```python
from build123d import *

# Parameters (mm, degrees)
SKETCH_1_W               = 20
SKETCH_1_H               = 10
EXTRUDE_1_DEPTH          = 9
CUT_EXTRUDE_3_DEPTH      = 9
CUT_EXTRUDE_4_DEPTH      = 18.52868966
CUT_EXTRUDE_4_DEPTH_BACK = 9
EXTRUDE_2_DEPTH          = 9
EXTRUDE_3_DEPTH          = 9
SKETCH_10_W              = 8
SKETCH_10_H              = 13
CUT_EXTRUDE_5_DEPTH      = 9
SKETCH_12_W              = 2.5
SKETCH_12_H              = 12
CUT_EXTRUDE_6_DEPTH      = 9
SKETCH_13_W              = 2.5
SKETCH_13_H              = 7.75
CUT_EXTRUDE_7_DEPTH      = 9
CUT_EXTRUDE_8_DEPTH      = 9
CUT_EXTRUDE_9_DEPTH      = 9
SKETCH_18_R              = 0.25
CUT_EXTRUDE_12_DEPTH     = 18.568302001
SKETCH_26_R              = 0.25
CUT_EXTRUDE_16_DEPTH     = 19.638541659


with BuildPart() as part:
    # 草图1 → 凸台-拉伸1 (new body)
    with BuildSketch(Plane(origin=(0, 0, 0), x_dir=(0, 0, -1), z_dir=(1, 0, 0))):
        with Locations((-3.964524465, 0.58990319)):
            Rectangle(SKETCH_1_W, SKETCH_1_H)
    extrude(amount=EXTRUDE_1_DEPTH)

    # 草图2 → 切除-拉伸3 (cut)
    with BuildSketch(Plane(origin=(9, 0, 0), x_dir=(0, 0, -1), z_dir=(1, 0, 0))):
        Polygon((0.035475535, -0.41009681), (-3.964524465, -4.41009681), (6.035475535, -4.41009681), (6.035475535, -0.410096535), align=None)
    extrude(amount=-CUT_EXTRUDE_3_DEPTH, mode=Mode.SUBTRACT)

    # 草图6 → 切除-拉伸4 (cut, two sides: drawn at the far end of the back side and taken through both)
    with BuildSketch(Plane(origin=(9, 0, 0), x_dir=(0, 0, -1), z_dir=(1, 0, 0)).offset(-CUT_EXTRUDE_4_DEPTH_BACK)):
        Polygon((-66.684543288, -0.910096672), (-13.964524465, -0.910096672), (-3.964524465, -0.910096672), (0.035475535, 3.089903328), (6.035475535, 3.089903328), (58.755494358, 3.089903328), (55.394957379, 108.476374614), (-70.045080267, 104.476374614), align=None)
    extrude(amount=CUT_EXTRUDE_4_DEPTH + CUT_EXTRUDE_4_DEPTH_BACK, mode=Mode.SUBTRACT)

    # 草图8 → 凸台-拉伸2 (add)
    with BuildSketch(Plane(origin=(9, 0, 0), x_dir=(0, 0, -1), z_dir=(1, 0, 0))):
        with BuildLine():
            Line((-13.964524465, -4.41009681), (-13.964524465, -0.910096672))
            ThreePointArc((-13.964524465, -0.910096672), (-15.714524534, -2.660096741), (-13.964524465, -4.41009681))
        make_face()
    extrude(amount=-EXTRUDE_2_DEPTH)

    # 草图9 → 凸台-拉伸3 (add)
    with BuildSketch(Plane(origin=(9, 0, 0), x_dir=(0, 0, -1), z_dir=(1, 0, 0))):
        with BuildLine():
            Line((6.035475535, -0.410096672), (6.035475535, 3.089903328))
            ThreePointArc((6.035475535, 3.089903328), (7.785475535, 1.339903328), (6.035475535, -0.410096672))
        make_face()
    extrude(amount=-EXTRUDE_3_DEPTH)

    # 草图10 → 切除-拉伸5 (cut)
    with BuildSketch(Plane(origin=(0, -0.910096672, 0), x_dir=(1, 0, 0), z_dir=(0, 1, 0))):
        with Locations((4.5, -10.464524465)):
            Rectangle(SKETCH_10_W, SKETCH_10_H)
    extrude(amount=-CUT_EXTRUDE_5_DEPTH, mode=Mode.SUBTRACT)

    # 草图12 → 切除-拉伸6 (cut)
    with BuildSketch(Plane(origin=(0, 3.089903328, 0), x_dir=(1, 0, 0), z_dir=(0, 1, 0))):
        with Locations((7.75, 6.035475535)):
            Rectangle(SKETCH_12_W, SKETCH_12_H)
    extrude(amount=-CUT_EXTRUDE_6_DEPTH, mode=Mode.SUBTRACT)

    # 草图13 → 切除-拉伸7 (cut)
    with BuildSketch(Plane(origin=(0, 3.089903328, 0), x_dir=(1, 0, 0), z_dir=(0, 1, 0))):
        with Locations((1.25, 3.910475535)):
            Rectangle(SKETCH_13_W, SKETCH_13_H)
    extrude(amount=-CUT_EXTRUDE_7_DEPTH, mode=Mode.SUBTRACT)

    # 草图14 → 切除-拉伸8 (cut)
    with BuildSketch(Plane(origin=(0, 1.527213896, 1.527213896), x_dir=(1, 0, 0), z_dir=(0, 0.7071067811865477, 0.7071067811865475))):
        Polygon((2.5, 2.209976588), (0, -3.446877662), (-6.872938914, -0.617067375), (-4.372938914, 5.039786874), align=None)
    extrude(amount=-CUT_EXTRUDE_8_DEPTH, mode=Mode.SUBTRACT)

    # 草图15 → 切除-拉伸9 (cut)
    with BuildSketch(Plane(origin=(0, 1.527213896, 1.527213896), x_dir=(1, 0, 0), z_dir=(0, 0.7071067811865477, 0.7071067811865475))):
        Polygon((6.5, 2.209976588), (9, -3.446877662), (12.673354488, 0), (10.173354488, 5.656854249), align=None)
    extrude(amount=-CUT_EXTRUDE_9_DEPTH, mode=Mode.SUBTRACT)

    # 草图18 → 切除-拉伸12 (cut, through all)
    with BuildSketch(Plane(origin=(6.5, 0, 0), x_dir=(0, 0, -1), z_dir=(1, 0, 0))):
        with Locations((6.035475535, 1.339903328)):
            Circle(SKETCH_18_R)
    extrude(amount=-CUT_EXTRUDE_12_DEPTH, mode=Mode.SUBTRACT)

    # 草图26 → 切除-拉伸16 (cut, through all)
    with BuildSketch(Plane.ZY):
        with Locations((13.964524465, -2.660096741)):
            Circle(SKETCH_26_R)
    extrude(amount=-CUT_EXTRUDE_16_DEPTH, mode=Mode.SUBTRACT)


solid = part.part
```
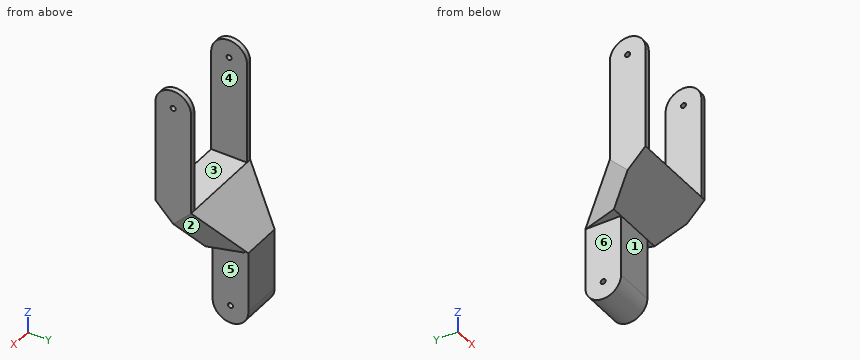
Part model, mm, in its own coordinate system. Face numbers are marked on the shaded views. A direction names the side the tool comes from. Round coordinates to 2 decimals unless told otherwise and drop trailing zeros. Loops run counter-clockwise (first coordinate to the right, second up) from the corner with the lowest first, then second, coordinate; pieces in that order, holes last. Notation, with made-up numbers: (24, -9) -> (66, -9) arc R23 cw to (66, 18) -> close; hole circle Ø2 at (-36, -32.5). An arc over 180 degrees is marked (long way). Use CSV: the item, a comma, the result in double quotes. Start each with the question number.
1) Cut at A-A, the plane z = 6. Write the cut outline in (x, y).
2) Cut at B-B, the plane x = 2.75. Write the cut outline in (y, z).
3) Which spindle directions (+Z, -Z, +X, -X, +Y, -Y) get a long thin tool onto all of the face, cutting with end or side? Do the marked faces 4, 5 and 6. Say none if no direction does.
4) Wall check: L1, parallel to X at y = -3.75, z = 11.5; L2, parallel to Y at x = 4.5, z = -3.5; L3, parallel to X at y = -0.5, z = 3.5. Give the ranges that are in metal, low to high. Write a range as [from, to].
5) Cut at D-D, the plane x = 6.75. Write the cut outline in (y, z), plus the area to 3 significant figures.
6) Pull direction X, two halves, no side cores. Call the marked faces 1, 2 and 3: +X half, -X half, draft (parallel to the pull), parting line (faces both ways), or undercut.
7) Drop flat-ended pins along their axis: P1, Ø2, axis at x = 4.5, z = -3, coming from the -Y side; P2, Ø0.9, axis at x = 7, y = 1, coming from the -Z side; P3, Ø1, axis at x = 2.5, y = 0.5, coming from the -Z side. Give the stop position or say it passes through.
8) Cut at C-C, the plane y = 0. Write the cut outline in (x, z).
Determined:
1,outline,"(0, -4.41) -> (0.5, -4.41) -> (0.5, -0.91) -> (0, -0.91) -> close; (8.5, -4.41) -> (9, -4.41) -> (9, -0.91) -> (8.5, -0.91) -> close"
2,outline,"(-4.41, 3.96) -> (-0.41, -0.04) -> (-0.41, -6.04) arc R1.75 ccw to (3.09, -6.04) -> (3.09, -0.04) -> (-0.91, 3.96) -> close; hole circle Ø0.5 at (1.34, -6.04)"
3,face 4,"+Z, +Y, -Y"
3,face 5,"-Z, +X, +Y, -Y"
3,face 6,"-Z, -X, +Y, -Y"
4,L1,"x = [0, 0.5], [8.5, 9]"
4,L2,"y = [-0.41, 3.09]"
4,L3,"x = [0.27, 8.73]"
5,outline,"(-4.41, 3.96) -> (-0.41, -0.04) -> (2.29, -0.04) -> (2.69, 0.36) -> (-0.91, 3.96) -> close"
5,area,"13.8 mm2"
6,face 1,"draft"
6,face 2,"+X half"
6,face 3,"undercut"
7,P1,"stops at y = -0.41"
7,P2,"stops at z = -0.04"
7,P3,"stops at z = -7.75"
8,outline,"(0.57, 3.05) -> (1.53, -0.04) -> (2.5, -0.04) -> (2.5, -7.16) -> (6.5, -7.16) -> (6.5, -0.04) -> (7.47, -0.04) -> (8.43, 3.05) -> close"
